Could you check a few things on this model? Use its own coordinates, in mm. A direction names the side the tool comes from. Coordinates: 2 decimals unless noted, no trailing zeros. Loops run counter-clockwise (first coordinate to the right, second up) from the corner with the lowest first, then second, coordinate; pieces in that order, holes last.
from build123d import *

# Parameters (mm, degrees)
CHAMFER1_SIZE  = 1.5
CHAMFER1_SIZE2 = 2.598076211


with BuildPart() as part:
    # Sketch1 → Revolve1 (revolve)
    with BuildSketch(Plane.XY):
        Polygon((5.05, -18.56), (5.05, 18.56), (9.5, 18.56), (9.5, 15.56), (11.5, 15.56), (11.5, -15.56), (9.5, -15.56), (9.5, -18.56), (9.5, -21.56), (6.3, -27.102562584), (5.05, -27.102562584), align=None)
    revolve(axis=Axis((0, 19.533170402, 0), (0, -1, 0)))

    # Chamfer1
    chamfer1_edges = [part.edges().sort_by_distance(p)[0] for p in [
        (-5.05, 18.56, 0),
    ]]
    chamfer1_side = [part.faces().sort_by_distance(p)[0] for p in [
        (-5.318700577, 18.56, 0),
    ]]
    chamfer(chamfer1_edges, length=CHAMFER1_SIZE, length2=CHAMFER1_SIZE2, reference=chamfer1_side[0])


solid = part.part
1) We'd pull the mould along X, two halves only. Please class faces 1 (the cylindrical face through (4.817, -5.872, 1.517)), 2 (the flat face through (4, 15.56, 9)), 3 (the conical face through (6.16, -26.83, 1.94)): released by +X, released by -X, zero draft, split by the parting line, or undercut.
2) Imagine slicing it at C-C on y = 10.5. List the corners of the cut face in (x, z) for me.
3) If I drill on L1, parallel to Z at x = 0, y = -11.5; L2, parallel to Y at x = 8.5, z = 5.5; L3, parallel to X at y = -15.5, z = 4, over which ranges is the centre line in solid material (lowest first)?
4) Imagine slicing it at A-A on x = 0. List the corners of the cut face in (y, z) for me.
5) For faces 4 (the flat face through (-2, 18.56, 6.5)), 5 (the cylindrical face through (4.38, -18.52, -8.43)), 6 (the cylindrical face through (4.38, 17.04, -8.43)), which set-ups out of +Z, -Z, +X, -X, +Y, -Y let a thin tool reach every point of the face, with its end or its side?
6) Will these pins go through, and if not, where does the flat tip stop? pin 1 (8 mm diameter, centred on y = -21.5, z = 3.5, fed in from -X); pin 2 (8 mm diameter, centred on x = 5.5, z = -8, fed in from +Y); pin 3 (2 mm diameter, centred on x = -4, y = -6, fed in from +Z); pin 4 (5 mm diameter, centred on y = 9.5, z = -3, fed in from -X).
7) Imagine slicing it at B-B on z = 0. List the corners of the cut face in (x, y) for me, plus the area to 3 significant figures.
Solved:
1. face 1: undercut
1. face 2: zero draft
1. face 3: split by the parting line
2. outline: circle Ø23 at (0, 0); hole circle Ø10.1 at (0, 0)
3. L1: z = -11.5 to -5.05, 5.05 to 11.5
3. L2: y = -15.56 to 15.56
3. L3: x = -10.78 to -3.08, 3.08 to 10.78
4. outline: (-27.1, -6.3) - (-21.56, -9.5) - (-15.56, -9.5) - (-15.56, -11.5) - (15.56, -11.5) - (15.56, -9.5) - (18.56, -9.5) - (18.56, -6.55) - (15.96, -5.05) - (-27.1, -5.05) - close; (-27.1, 5.05) - (15.96, 5.05) - (18.56, 6.55) - (18.56, 9.5) - (15.56, 9.5) - (15.56, 11.5) - (-15.56, 11.5) - (-15.56, 9.5) - (-21.56, 9.5) - (-27.1, 6.3) - close
5. face 4: +Z, -Z, +X, -X, +Y
5. face 5: -Y
5. face 6: +Y
6. pin 1: stops at x = -9.5
6. pin 2: stops at y = 18.56
6. pin 3: stops at z = 11.1
6. pin 4: stops at x = -11.49
7. outline: (-11.5, -15.56) - (-9.5, -15.56) - (-9.5, -21.56) - (-6.3, -27.1) - (-5.05, -27.1) - (-5.05, 15.96) - (-6.55, 18.56) - (-9.5, 18.56) - (-9.5, 15.56) - (-11.5, 15.56) - close; (5.05, -27.1) - (6.3, -27.1) - (9.5, -21.56) - (9.5, -15.56) - (11.5, -15.56) - (11.5, 15.56) - (9.5, 15.56) - (9.5, 18.56) - (6.55, 18.56) - (5.05, 15.96) - close
7. area: 509 mm2
